Read the model definition and answer for the solid it produces. Units are mm, in the model's axes. A direction names the side the tool comes from. Give positions to 0.01 mm unless a question says otherwise; leave off trailing zeros. Loops run counter-clockwise (first coordinate to the right, second up) from the corner with the lowest first, then second, coordinate; pieces in that order, holes last.
(1) Find section C-C, the plane y = 3.25. Write down the section's boundary in (x, z), then the cut area to 3 significant figures.
(2) Find section D-D, the plane x = -6. Write down the section's boundary in (y, z), then the cut area to 3 significant figures.
(3) Determine the mould class of faces 6 (the face through (0.42, -1.88, -0.33)), 7 (the face through (-7.648, 0.513, 7.972)), 8 (the face through (7.648, -0.513, 7.972)), 9 (the face through (6.87, 3.4, 7.97)) for opening direction X: pulls with the +X half, pulls with the -X half, needs draft (parallel to the pull), parting line crosses it, or undercut.
(4) Find section A-A, the plane y = 6.25. Write down the section's boundary in (x, z), then the cut area to 3 significant figures.
(5) Which of the six approach directions +Z, -Z, +X, -X, +Y, -Y give full straight-line access (tool end or side, diameter ignored) to faces 1 (the face through (-2.45, 7.26, 7.97)), 2 (the face through (-7.26, 2.45, 7.97)), 3 (the face through (7.26, -2.45, 7.97)), 4 (the face through (3.4, 6.87, 7.97)), 5 (the face through (-0.513, -7.648, 7.972))?
(6) Straight lines are drawn through the part: probe 1 along X at (y, z) = (8.5, 9); probe 2 along Z at (x, y) = (-3, 3.75). For each, find the intervals that lie inside material, in ascending order.
(7) Each of these flat-tipped pins is pushed along its axis until it touches: P1, Ø5, axis at y = 4, z = -1.5, coming from the +X side; P2, Ø3, axis at x = 7.5, z = 6, coming from the +Y side. Where does it stop, or does it pass through?
Autodesk Inventor part; units mm, degrees
ref_plane "YZ Plane" through (0, 0, 0) normal (1, 0, 0) x (0, 1, 0)
ref_plane "XZ Plane" through (0, 0, 0) normal (0, 1, 0) x (-1, 0, 0)
ref_plane "XY Plane" through (0, 0, 0) normal (0, 0, 1) x (1, 0, 0)
sketch "Szkic1" plane through (0, 0, 0) normal (0, 0, 1) x (1, 0, 0)
  circle A0 centre (0, 0) radius 3.25
  dimension "d0" = 6.5
extrude "Wyciągnięcie proste1" add sketch "Szkic1" along normal blind 6
sketch "Szkic3" plane through (0, 0, 0) normal (0, 0, -1) x (-1, 0, 0)
  circle A0 centre (0, 0) radius 3.65
  dimension "d11" = 7.3
extrude "Wyciągnięcie proste3" add sketch "Szkic3" against normal blind 6
sketch "Szkic4" plane through (0, 0, 6) normal (0, 0, 1) x (1, 0, 0)
  circle A0 centre (0, 0) radius 3.65
  circle A1 centre (0, 0) radius 3.65
  line L0 (0, 0) -> (0, 9)
  line L1 (0, 9) -> (0, 9.5)
  line L2 (0, 9.5) -> (6.3185, 9.5) construction
  line L3 (0, 9.5) -> (0, 10)
  line L4 (0, 10) -> (1.4493, 3.3499)
  line L5 (0, 10) -> (-1.4493, 3.3499)
  line L6 (-3.8268, 9.2388) -> (0.057, 3.6496)
  line L7 (-3.8268, 9.2388) -> (-2.6209, 2.5403)
  line L8 (-7.0711, 7.0711) -> (-1.344, 3.3936)
  line L9 (-7.0711, 7.0711) -> (-3.3936, 1.344)
  line L10 (-9.2388, 3.8268) -> (-2.5403, 2.6209)
  line L11 (-9.2388, 3.8268) -> (-3.6496, -0.057)
  line L12 (-10, 0) -> (-3.3499, 1.4493)
  line L13 (-10, 0) -> (-3.3499, -1.4493)
  line L14 (-9.2388, -3.8268) -> (-3.6496, 0.057)
  line L15 (-9.2388, -3.8268) -> (-2.5403, -2.6209)
  line L16 (-7.0711, -7.0711) -> (-3.3936, -1.344)
  line L17 (-7.0711, -7.0711) -> (-1.344, -3.3936)
  line L18 (-3.8268, -9.2388) -> (-2.6209, -2.5403)
  line L19 (-3.8268, -9.2388) -> (0.057, -3.6496)
  line L20 (0, -10) -> (-1.4493, -3.3499)
  line L21 (0, -10) -> (1.4493, -3.3499)
  line L22 (3.8268, -9.2388) -> (-0.057, -3.6496)
  line L23 (3.8268, -9.2388) -> (2.6209, -2.5403)
  line L24 (7.0711, -7.0711) -> (1.344, -3.3936)
  line L25 (7.0711, -7.0711) -> (3.3936, -1.344)
  line L26 (9.2388, -3.8268) -> (2.5403, -2.6209)
  line L27 (9.2388, -3.8268) -> (3.6496, 0.057)
  line L28 (10, 0) -> (3.3499, -1.4493)
  line L29 (10, 0) -> (3.3499, 1.4493)
  line L30 (9.2388, 3.8268) -> (3.6496, -0.057)
  line L31 (9.2388, 3.8268) -> (2.5403, 2.6209)
  line L32 (7.0711, 7.0711) -> (3.3936, 1.344)
  line L33 (7.0711, 7.0711) -> (1.344, 3.3936)
  line L34 (3.8268, 9.2388) -> (2.6209, 2.5403)
  line L35 (3.8268, 9.2388) -> (-0.057, 3.6496)
  point P0 (-2.9615, 4.4322)
  point P1 (-4.4322, 2.9615)
  point P2 (-5.2282, 1.0399)
  point P3 (-5.2282, -1.0399)
  point P4 (-4.4322, -2.9615)
  point P5 (-2.9615, -4.4322)
  point P6 (-1.0399, -5.2282)
  point P7 (1.0399, -5.2282)
  point P8 (2.9615, -4.4322)
  point P9 (4.4322, -2.9615)
  point P10 (5.2282, -1.0399)
  point P11 (5.2282, 1.0399)
  point P12 (4.4322, 2.9615)
  point P13 (2.9615, 4.4322)
  point P14 (1.0399, 5.2282)
  point P15 (-1.0399, 5.2282)
  dimension "d34" = 9
  dimension "d39" = 0.5
  dimension "d49" = 0.5
  dimension "d52" = 360
extrude "Wyciągnięcie proste4" add sketch "Szkic4" along normal blind 4
sketch "Szkic5" plane through (0, 0, 0) normal (0, 0, -1) x (-1, 0, 0)
  circle A0 centre (0, 0) radius 3.65
extrude "Wyciągnięcie proste5" add sketch "Szkic5" along normal blind 6
sketch "Szkic6" plane through (0, 0, -6) normal (0, 0, -1) x (-1, 0, 0)
  circle A0 centre (0, 0) radius 1.425
  circle A1 centre (0, 0) radius 3.65
  dimension "d30" = 2.85
extrude "Wyciągnięcie proste6" cut sketch "Szkic6" against normal blind 12
fillet "Zaokrąglenie1" radius 0.5 1 edges at (1.425, 0, 6)
sketch "Szkic7" plane through (0, 0, -6) normal (0, 0, -1) x (-1, 0, 0)
  circle A0 centre (0, 0) radius 1.925
  dimension "d45" = 3.85
extrude "Wyciągnięcie proste7" add sketch "Szkic7" against normal blind 12.75
fillet "Zaokrąglenie2" radius 0.5 1 edges at (1.925, 0, 6)
properties part number "GEAR"
Entries:
1. outline: (-8.41, 6) - (-6.03, 6) - (-6.03, 10) - (-8.41, 10) - close; (-4.62, 6) - (4.62, 6) - (4.62, 10) - (-4.62, 10) - close; (6.03, 6) - (8.41, 6) - (8.41, 10) - (6.03, 10) - close
1. area: 55.9 mm2
2. outline: (-6.38, 6) - (-5.4, 6) - (-5.4, 10) - (-6.38, 10) - close; (-3.24, 6) - (-1.58, 6) - (-1.58, 10) - (-3.24, 10) - close; (-0.87, 6) - (0.87, 6) - (0.87, 10) - (-0.87, 10) - close; (1.58, 6) - (3.24, 6) - (3.24, 10) - (1.58, 10) - close; (5.4, 6) - (6.38, 6) - (6.38, 10) - (5.4, 10) - close
2. area: 28.2 mm2
3. face 6: parting line crosses it
3. face 7: pulls with the -X half
3. face 8: pulls with the +X half
3. face 9: undercut
4. outline: (-6.54, 6) - (-5.79, 6) - (-5.79, 10) - (-6.54, 10) - close; (-3.29, 6) - (-1.75, 6) - (-1.75, 10) - (-3.29, 10) - close; (-0.82, 6) - (0.82, 6) - (0.82, 10) - (-0.82, 10) - close; (1.75, 6) - (3.29, 6) - (3.29, 10) - (1.75, 10) - close; (5.79, 6) - (6.54, 6) - (6.54, 10) - (5.79, 10) - close
4. area: 24.9 mm2
5. face 1: +Z, -Z, +Y
5. face 2: +Z, -Z, -X
5. face 3: +Z, -Z, +X
5. face 4: +Z, -Z
5. face 5: +Z, -Z, -Y
6. probe 1: x = -3.69 to -3.31, -0.33 to 0.33, 3.31 to 3.69
6. probe 2: z = 6 to 10
7. P1: stops at x = 1.21
7. P2: stops at y = 7.07
